Can you work these out from the model? Positions are in its coordinate system, mm. A direction names the side the tool comes from. Coordinates: 2 decimals unless noted, no trailing zeros. Loops run counter-clockwise (first coordinate to the right, second up) from the corner with the lowest first, then second, coordinate; pieces in that order, holes last. Notation, with made-up numbers: (-11, 56) -> (-1, 56) arc R23 cw to (-1, 95) -> close; hole circle Ø10 at (-36, -31.5). An arc over 180 degrees is marked (long way). Put each result on its own line as item: value. Start each with the question number.
Item 1: If we section it at D-D on y = -35.5: Please give me the cut outline in (x, z), plus the area to 4 significant figures.
Item 2: Please list where these lines run through material, in increasing order: L1, parallel to Z at x = 17.5, y = 2; L2, parallel to X at y = -6, z = -94; L3, parallel to Y at x = 25.75, z = -16. Write a range as from..to.
Item 3: If we section it at A-A on y = -20: Please give me the cut outline in (x, z), plus the area to 3 significant figures.
Item 4: Will these pins go through, and if not, where does the flat tip stop? P1, Ø8, axis at x = 20.5, y = -16, coming from the -Z side; P2, Ø1.5, axis at x = 13.5, z = -66.5, coming from the +Y side; P3, Ø7.5, axis at x = 18, y = -25, coming from the +Z side.
Item 5: If we section it at C-C on y = 2.5: Please give me the cut outline in (x, z), plus the area to 3 significant figures.
Item 6: We'd pull the mould along X, two halves only. Please class faces 5 (the flat face through (15, 4, -61)), 6 (the flat face through (27.5, -15, -82)), 7 (the cylindrical face through (2.85, 4.06, -116.99)): pulls with the +X half, pulls with the -X half, needs draft (parallel to the pull), parting line crosses it, or undercut.
Item 7: If we section it at B-B on x = 15: Please give me the cut outline in (y, z), plus the area to 3 significant figures.
Item 8: For faces 1 (the flat face through (15, 6, -20)), 2 (the flat face through (15, -11, -100)), 3 (the flat face through (2.5, -11, -86)), 4 (the flat face through (15, 4, -120)), which set-ups out of +Z, -Z, +X, -X, +Y, -Y let a thin tool reach every point of the face, with its end or its side?
```python
from build123d import *

# Parameters (mm, degrees)
SKETCH1_W           = 30
SKETCH1_H           = 120
BOSS_EXTRUDE1_DEPTH = 8
SKETCH2_W           = 30
SKETCH2_H           = 80
CUT_EXTRUDE1_DEPTH  = 4
SKETCH3_W           = 30
SKETCH3_H           = 3
BOSS_EXTRUDE2_DEPTH = 40
SKETCH4_R           = 8.6
CUT_EXTRUDE2_DEPTH  = 40
BOSS_EXTRUDE3_DEPTH = 2.5
BOSS_EXTRUDE4_DEPTH = 2.5
SKETCH7_R           = 3
CUT_EXTRUDE3_DEPTH  = 131
FILLET1_R           = 10


with BuildPart() as part:
    # Sketch1 → Boss-Extrude1 (new body)
    with BuildSketch(Plane(origin=(0, 0, 0), x_dir=(1, 0, 0), z_dir=(0, 1, 0))):
        with Locations((15, 60)):
            Rectangle(SKETCH1_W, SKETCH1_H)
    extrude(amount=BOSS_EXTRUDE1_DEPTH)

    # Sketch2 → Cut-Extrude1 (cut)
    with BuildSketch(Plane(origin=(0, 8, 0), x_dir=(1, 0, 0), z_dir=(0, 1, 0))):
        with Locations((15, 60)):
            Rectangle(SKETCH2_W, SKETCH2_H)
    extrude(amount=-CUT_EXTRUDE1_DEPTH, mode=Mode.SUBTRACT)

    # Sketch3 → Boss-Extrude2 (add)
    with BuildSketch(Plane.XZ):
        with Locations((15, -98.5)):
            Rectangle(SKETCH3_W, SKETCH3_H)
    extrude(amount=BOSS_EXTRUDE2_DEPTH)

    # Sketch4 → Cut-Extrude2 (cut)
    with BuildSketch(Plane.XY.offset(-97)):
        with Locations((15, -20)):
            Circle(SKETCH4_R)
    extrude(amount=-CUT_EXTRUDE2_DEPTH, mode=Mode.SUBTRACT)

    # Sketch5 → Boss-Extrude3 (add)
    with BuildSketch(Plane(origin=(30, 0, 0), x_dir=(0, 0, -1), z_dir=(1, 0, 0))):
        Polygon((97, -40), (57, 0), (97, 0), align=None)
    extrude(amount=-BOSS_EXTRUDE3_DEPTH)

    # Sketch6 → Boss-Extrude4 (add)
    with BuildSketch(Plane.ZY):
        Polygon((-57, 0), (-97, -40), (-97, 0), align=None)
    extrude(amount=-BOSS_EXTRUDE4_DEPTH)

    # Sketch7 → Cut-Extrude3 (cut, through all)
    with BuildSketch(Plane(origin=(0, 0, 0), x_dir=(-1, 0, 0), z_dir=(0, -1, 0))):
        with Locations(Location((-15, 10, 0), (0, 0, 90))):
            Circle(SKETCH7_R)
        with Locations(Location((-15, 110, 0), (0, 0, 90))):
            Circle(SKETCH7_R)
    extrude(amount=-CUT_EXTRUDE3_DEPTH, mode=Mode.SUBTRACT)

    # Fillet1
    fillet1_edges = [part.edges().sort_by_distance(p)[0] for p in [
        (0, 4, -120),
        (30, 4, -120),
        (30, 4, 0),
        (0, 4, 0),
    ]]
    fillet(fillet1_edges, radius=FILLET1_R)


solid = part.part
```
Solutions:
1. outline: (0, -100) -> (30, -100) -> (30, -92.5) -> (27.5, -92.5) -> (27.5, -97) -> (2.5, -97) -> (2.5, -92.5) -> (0, -92.5) -> close
1. area: 112.5 mm^2
2. L1: -120..-111.66, -108.34..-11.66, -8.34..0
2. L2: 0..2.5, 27.5..30
2. L3: 0..8
3. outline: (0, -100) -> (6.4, -100) -> (6.4, -97) -> (2.5, -97) -> (2.5, -77) -> (0, -77) -> close; (23.6, -100) -> (30, -100) -> (30, -77) -> (27.5, -77) -> (27.5, -97) -> (23.6, -97) -> close
3. area: 138 mm^2
4. P1: z = -100
4. P2: y = 4
4. P3: z = -97
5. outline: (0, -110) arc R10 ccw to (10, -120) -> (20, -120) arc R10 ccw to (30, -110) -> (30, -10) arc R10 ccw to (20, 0) -> (10, 0) arc R10 ccw to (0, -10) -> close; hole circle Ø6 at (15, -110); hole circle Ø6 at (15, -10)
5. area: 3,460 mm^2
6. face 5: needs draft
6. face 6: undercut
6. face 7: pulls with the -X half
7. outline: (-40, -100) -> (-28.6, -100) -> (-28.6, -97) -> (-40, -97) -> close; (-11.4, -100) -> (0, -100) -> (0, -107) -> (8, -107) -> (8, -100) -> (4, -100) -> (4, -20) -> (8, -20) -> (8, -13) -> (0, -13) -> (0, -97) -> (-11.4, -97) -> close; (0, -120) -> (8, -120) -> (8, -113) -> (0, -113) -> close; (0, -7) -> (8, -7) -> (8, 0) -> (0, 0) -> close
7. area: 612 mm^2
8. face 1: +X, -X, +Y
8. face 2: -Z, +X, -X, -Y
8. face 3: +Z, -Y
8. face 4: -Z, +X, -X, +Y, -Y
